Could you check a few things on this model? Use its own coordinates, in mm. Face numbers are marked on the shaded views. A direction names the side the tool comes from. Coordinates: 2 decimals unless noted, no trailing zeros. Loops run counter-clockwise (first coordinate to the right, second up) from the corner with the lowest first, then second, coordinate; pieces in that order, holes last. Notation, with made-up numbers: (-35.5, -24) - (-3.5, -24) arc R8 cw to (-3.5, -16) - close; hole circle Ø3 at (46.25, 71.25). An arc over 180 degrees is marked (long way). One line per question, with ' | ' between items. Start each with the question number.
1. I'm going to push flat-ended pins straight in: P1, Ø1.3, axis at y = 1.5, z = 18, coming from the -X side; P2, Ø2, axis at y = 0.5, z = 4, coming from the +X side; P3, Ø0.8, axis at y = 2.5, z = -17.5, coming from the +X side. Where does each tip first touch, or does it pass through?
2. I want a section at D-D, the plane z = -16. Write out the boundary of the cut face in (x, y), then the cut area to 3 significant figures.
3. I want a section at A-A, the plane z = 0. Write out the boundary of the cut face in (x, y), then the cut area to 3 significant figures.
4. I want a section at B-B, the plane x = 0. Write out the boundary of the cut face in (y, z).
5. Which directions (+Z, -Z, +X, -X, +Y, -Y) give clear straight access to the entire face, cutting with the end or side of a thin tool? Please do the marked faces 1, 2 and 3.
6. We'd pull the mould along X, two halves only. Please class the marked faces 4, 5 and 6: pulls with the +X half, pulls with the -X half, needs draft (parallel to the pull), parting line crosses it, or undercut.
7. Please list where these lines run through material, in increasing order: L1, parallel to Z at x = 0, y = 2.25; L2, parallel to X at y = 1.5, z = 17; L3, parallel to X at y = 1.45, z = 11. Write a range as [from, to].
from build123d import *

# Parameters (mm, degrees)
SKETCH_2_R      = 13.75
EXTRUDE_1_DEPTH = 5


with BuildPart() as part:
    # Эскиз2 → Бобышка-Вытянуть1 (new body)
    with BuildSketch(Plane(origin=(0, 0, 0), x_dir=(1, 0, 0), z_dir=(0, 1, 0))):
        with BuildLine():
            Line((-2.85, 18.279154794), (-2.85, 16.657956057))
            ThreePointArc((-2.85, 16.657956057), (-6.467350007, 15.613564099), (-9.763699362, 13.794208015))
            Line((-9.763699362, 13.794208015), (-10.910059983, 14.940568636))
            ThreePointArc((-10.910059983, 14.940568636), (-13.081475452, 13.081475452), (-14.940568636, 10.910059983))
            Line((-14.940568636, 10.910059983), (-13.794208015, 9.763699362))
            ThreePointArc((-13.794208015, 9.763699362), (-15.613564099, 6.467350007), (-16.657956057, 2.85))
            Line((-16.657956057, 2.85), (-18.279154794, 2.85))
            ThreePointArc((-18.279154794, 2.85), (-18.5, 0), (-18.279154794, -2.85))
            Line((-18.279154794, -2.85), (-16.657956057, -2.85))
            ThreePointArc((-16.657956057, -2.85), (-15.613564099, -6.467350007), (-13.794208015, -9.763699362))
            Line((-13.794208015, -9.763699362), (-14.940568636, -10.910059983))
            ThreePointArc((-14.940568636, -10.910059983), (-13.081475452, -13.081475452), (-10.910059983, -14.940568636))
            Line((-10.910059983, -14.940568636), (-9.763699362, -13.794208015))
            ThreePointArc((-9.763699362, -13.794208015), (-6.467350007, -15.613564099), (-2.85, -16.657956057))
            Line((-2.85, -16.657956057), (-2.85, -18.279154794))
            ThreePointArc((-2.85, -18.279154794), (0, -18.5), (2.85, -18.279154794))
            Line((2.85, -18.279154794), (2.85, -16.657956057))
            ThreePointArc((2.85, -16.657956057), (6.467350007, -15.613564099), (9.763699362, -13.794208015))
            Line((9.763699362, -13.794208015), (10.910059983, -14.940568636))
            ThreePointArc((10.910059983, -14.940568636), (13.081475452, -13.081475452), (14.940568636, -10.910059983))
            Line((14.940568636, -10.910059983), (13.794208015, -9.763699362))
            ThreePointArc((13.794208015, -9.763699362), (15.613564099, -6.467350007), (16.657956057, -2.85))
            Line((16.657956057, -2.85), (18.279154794, -2.85))
            ThreePointArc((18.279154794, -2.85), (18.5, 0), (18.279154794, 2.85))
            Line((18.279154794, 2.85), (16.657956057, 2.85))
            ThreePointArc((16.657956057, 2.85), (15.613564099, 6.467350007), (13.794208015, 9.763699362))
            Line((13.794208015, 9.763699362), (14.940568636, 10.910059983))
            ThreePointArc((14.940568636, 10.910059983), (13.081475452, 13.081475452), (10.910059983, 14.940568636))
            Line((10.910059983, 14.940568636), (9.763699362, 13.794208015))
            ThreePointArc((9.763699362, 13.794208015), (6.467350007, 15.613564099), (2.85, 16.657956057))
            Line((2.85, 16.657956057), (2.85, 18.279154794))
            ThreePointArc((2.85, 18.279154794), (0, 18.5), (-2.85, 18.279154794))
        make_face()
        Circle(SKETCH_2_R, mode=Mode.SUBTRACT)
    extrude(amount=EXTRUDE_1_DEPTH)


solid = part.part
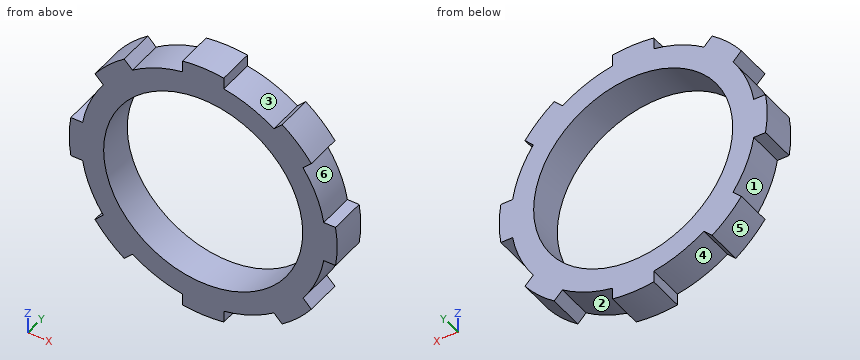
Results are:
1) P1: stops at x = -2.85 | P2: stops at x = 16.63 | P3: stops at x = 2.85
2) outline: (-5.44, 0) - (5.44, 0) - (5.44, 5) - (-5.44, 5) - close | area: 54.4 mm2
3) outline: (-18.5, 0) - (-13.75, 0) - (-13.75, 5) - (-18.5, 5) - close; (13.75, 0) - (18.5, 0) - (18.5, 5) - (13.75, 5) - close | area: 47.5 mm2
4) outline: (0, -18.5) - (5, -18.5) - (5, -13.75) - (0, -13.75) - close; (0, 13.75) - (5, 13.75) - (5, 18.5) - (0, 18.5) - close
5) face 1: -X, +Y, -Y | face 2: -Z, +Y, -Y | face 3: +Z, +Y, -Y
6) face 4: undercut | face 5: pulls with the -X half | face 6: pulls with the +X half
7) L1: z = [-18.5, -13.75], [13.75, 18.5] | L2: x = [-2.85, 2.85] | L3: x = [-14.87, -8.25], [8.25, 14.87]
